```python
from build123d import *

# Parameters (mm, degrees)
SKETCH1_W           = 13.5
SKETCH1_H           = 9.5
BOSS_EXTRUDE1_DEPTH = 9
SKETCH2_W           = 16
SKETCH2_H           = 12
BOSS_EXTRUDE2_DEPTH = 1.2
SKETCH3_R           = 1.4
CUT_EXTRUDE1_DEPTH  = 5
FILLET1_R           = 2
FILLET2_R           = 2
FILLET3_R           = 0.4
FILLET4_R           = 1


with BuildPart() as part:
    # Sketch1 → Boss-Extrude1 (new body)
    with BuildSketch(Plane.XY):
        Rectangle(SKETCH1_W, SKETCH1_H)
    extrude(amount=BOSS_EXTRUDE1_DEPTH)

    # Sketch2 → Boss-Extrude2 (add)
    with BuildSketch(Plane.XY.offset(9)):
        Rectangle(SKETCH2_W, SKETCH2_H)
    extrude(amount=BOSS_EXTRUDE2_DEPTH)

    # Sketch3 → Cut-Extrude1 (cut)
    with BuildSketch(Plane.XY.offset(10.2)):
        Circle(SKETCH3_R)
    extrude(amount=-CUT_EXTRUDE1_DEPTH, mode=Mode.SUBTRACT)

    # Fillet1
    fillet1_edges = [part.edges().sort_by_distance(p)[0] for p in [
        (6.75, -4.75, 4.5),
        (-6.75, -4.75, 4.5),
        (-6.75, 4.75, 4.5),
        (6.75, 4.75, 4.5),
    ]]
    fillet(fillet1_edges, radius=FILLET1_R)

    # Fillet2
    fillet2_edges = [part.edges().sort_by_distance(p)[0] for p in [
        (0, -4.75, 0),
        (6.75, 0, 0),
        (-6.75, 0, 0),
        (0, 4.75, 0),
        (-6.164213562, 4.164213562, 0),
        (6.164213562, 4.164213562, 0),
        (6.164213562, -4.164213562, 0),
        (-6.164213562, -4.164213562, 0),
    ]]
    fillet(fillet2_edges, radius=FILLET2_R)

    # Fillet3
    fillet3_edges = [part.edges().sort_by_distance(p)[0] for p in [
        (0, -4.75, 9),
        (-6.75, 0, 9),
        (6.75, 0, 9),
        (0, 4.75, 9),
        (-6.164213562, -4.164213562, 9),
        (6.164213562, -4.164213562, 9),
        (6.164213562, 4.164213562, 9),
        (-6.164213562, 4.164213562, 9),
    ]]
    fillet(fillet3_edges, radius=FILLET3_R)

    # Fillet4
    fillet4_edges = [part.edges().sort_by_distance(p)[0] for p in [
        (8, -6, 9.6),
        (8, 6, 9.6),
        (-8, 6, 9.6),
        (-8, -6, 9.6),
    ]]
    fillet(fillet4_edges, radius=FILLET4_R)


solid = part.part
```
Geometry: final body of the model. Coordinates: model frame, mm. A direction names the side the tool comes from. Give positions to 0.01 mm unless a question says otherwise; leave off trailing zeros. Order: outer loops, then holes, each group sorted by start corner. A loop starts at its lowest first (then second) coordinate and runs counter-clockwise, first axis right, second up. Notation, with made-up numbers: (-32.5, -14.5) -> (-23.5, -14.5) arc R27 cw to (-23.5, 1.5) -> close; hole circle Ø4 at (-9.75, 4.25). An arc over 180 degrees is marked (long way). Write each question's results on one line, items separated by ' | '. Start each with the question number.
1) Section D-D (y = 0). Return loops of the section in (x, z), then the cut area to 3 significant figures.
2) Section B-B (x = 4). Return loops of the section in (y, z).
3) Line query: line 1 (Y direction, x = 0, z = 6.55); line 2 (Y direction, x = 0, z = 9.1); line 3 (Y direction, x = -0.25, z = 2.5). Output: solid intervals per line, ascending. Write a range as from..to.
4) Section A-A (z = 8.25). Return loops of the section in (x, y).
5) Draft query along X for faces 4 (the flat face through (-6.75, 0, 5)), 5 (the cylindrical face through (-1.4, 0.06, 7.74)), 6 (the flat face through (0, 0, 5.2)), 7 (the cylindrical face through (-0.07, 4.18, 0.6)). Return one class per face: pulls with the +X half, pulls with the -X half, needs draft (parallel to the pull), parting line crosses it, or undercut.
6) Set-up query: faces 1 (the flat face through (-0.04, -5.31, 9)), 2 (the flat face through (6.75, 0, 5)), 3 (the flat face through (0, -4.75, 5)). Return all of +Z, -Z, +X, -X, +Y, -Y with unobstructed straight access to the full face (end or side cutting, diameter ignored); none if empty.
7) First-contact query: pin 1 (3 mm diameter, centred on y = 1, z = 6.5, fed in from +X); pin 2 (2 mm diameter, centred on x = -0.5, z = 6.5, fed in from -Y); pin 3 (2 mm diameter, centred on x = 0.5, z = 6, fed in from +Y). Flat tips, straight axial feed; report the tip coordinate or a pass-through.
8) Section C-C (z = 4.5). Return loops of the section in (x, y), then the cut area to 3 significant figures.
Calculated:
1) outline: (-8, 9) -> (-7.15, 9) arc R0.4 cw to (-6.75, 8.6) -> (-6.75, 2) arc R2 ccw to (-4.75, 0) -> (4.75, 0) arc R2 ccw to (6.75, 2) -> (6.75, 8.6) arc R0.4 cw to (7.15, 9) -> (8, 9) -> (8, 10.2) -> (1.4, 10.2) -> (1.4, 5.2) -> (-1.4, 5.2) -> (-1.4, 10.2) -> (-8, 10.2) -> close | area: 125 mm2
2) outline: (-6, 9) -> (-5.15, 9) arc R0.4 cw to (-4.75, 8.6) -> (-4.75, 2) arc R2 ccw to (-2.75, 0) -> (2.75, 0) arc R2 ccw to (4.75, 2) -> (4.75, 8.6) arc R0.4 cw to (5.15, 9) -> (6, 9) -> (6, 10.2) -> (-6, 10.2) -> close
3) line 1: -4.75..-1.4, 1.4..4.75 | line 2: -6..-1.4, 1.4..6 | line 3: -4.75..4.75
4) outline: (-6.75, -2.75) arc R2 ccw to (-4.75, -4.75) -> (4.75, -4.75) arc R2 ccw to (6.75, -2.75) -> (6.75, 2.75) arc R2 ccw to (4.75, 4.75) -> (-4.75, 4.75) arc R2 ccw to (-6.75, 2.75) -> close; hole circle Ø2.8 at (0, 0)
5) face 4: pulls with the -X half | face 5: undercut | face 6: undercut | face 7: needs draft
6) face 1: -Z | face 2: -Z, +X, +Y, -Y | face 3: -Z, +X, -X, -Y
7) pin 1: x = 6.75 | pin 2: y = -4.75 | pin 3: y = 4.75
8) outline: (-6.75, -2.75) arc R2 ccw to (-4.75, -4.75) -> (4.75, -4.75) arc R2 ccw to (6.75, -2.75) -> (6.75, 2.75) arc R2 ccw to (4.75, 4.75) -> (-4.75, 4.75) arc R2 ccw to (-6.75, 2.75) -> close | area: 125 mm2
